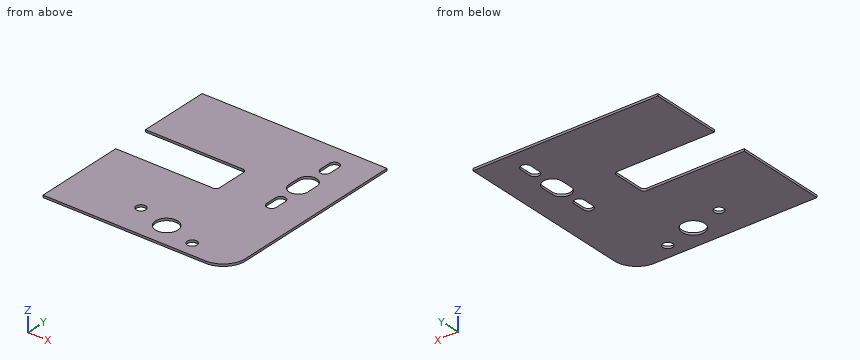
from build123d import *

# Parameters (mm, degrees)
ESQUISSE1_W             = 247
ESQUISSE1_H             = 267
ESQUISSE1_R             = 12.5
ESQUISSE1_R_2           = 6.5
BOSS_EXTRU_1_DEPTH      = 3
ESQUISSE3_R             = 6.5
ESQUISSE3_R_2           = 15
ENL_V_MAT_EXTRU_2_DEPTH = 3
ESQUISSE4_W             = 135
ESQUISSE4_H             = 50
ENL_V_MAT_EXTRU_3_DEPTH = 10
CONG_1_R                = 5
CONG_2_R                = 30
ENL_V_MAT_EXTRU_4_DEPTH = 10


with BuildPart() as part:
    # Esquisse1 → Boss.-Extru.1 (new body)
    with BuildSketch(Plane.XY):
        Rectangle(ESQUISSE1_W, ESQUISSE1_H)
        with Locations((76.5, 51.5)):
            Circle(ESQUISSE1_R, mode=Mode.SUBTRACT)
        with Locations((76.5, 96.5)):
            Circle(ESQUISSE1_R_2, mode=Mode.SUBTRACT)
        with Locations((76.5, 6.5)):
            Circle(ESQUISSE1_R_2, mode=Mode.SUBTRACT)
    extrude(amount=BOSS_EXTRU_1_DEPTH)

    # Esquisse3 → Enlèv. mat.-Extru.2 (cut)
    with BuildSketch(Plane(origin=(0, 0, 0), x_dir=(-1, 0, 0), z_dir=(0, 0, -1))):
        with Locations((-59.966662183, -113.5)):
            Circle(ESQUISSE3_R)
        with Locations((-16.5, -101.85314297)):
            Circle(ESQUISSE3_R_2)
        with Locations((26.966662183, -90.206285941)):
            Circle(ESQUISSE3_R)
    extrude(amount=-ENL_V_MAT_EXTRU_2_DEPTH, mode=Mode.SUBTRACT)

    # Esquisse4 → Enlèv. mat.-Extru.3 (cut)
    with BuildSketch(Plane(origin=(0, 0, 0), x_dir=(-1, 0, 0), z_dir=(0, 0, -1))):
        with Locations((56, 13.5)):
            Rectangle(ESQUISSE4_W, ESQUISSE4_H)
    extrude(amount=-ENL_V_MAT_EXTRU_3_DEPTH, mode=Mode.SUBTRACT)

    # Congé1
    cong_1_edges = [part.edges().sort_by_distance(p)[0] for p in [
        (11.5, -11.5, 1.5),
        (11.5, 38.5, 1.5),
    ]]
    fillet(cong_1_edges, radius=CONG_1_R)

    # Congé2
    cong_2_edges = [part.edges().sort_by_distance(p)[0] for p in [
        (123.5, -133.5, 1.5),
    ]]
    fillet(cong_2_edges, radius=CONG_2_R)

    # Esquisse5 → Enlèv. mat.-Extru.4 (cut)
    with BuildSketch(Plane(origin=(0, 0, 0), x_dir=(-1, 0, 0), z_dir=(0, 0, -1))):
        with BuildLine():
            Line((-83, 89), (-83, 104))
            ThreePointArc((-83, 104), (-76.5, 110.5), (-70, 104))
            Line((-70, 104), (-70, 89))
            ThreePointArc((-70, 89), (-76.5, 82.5), (-83, 89))
        make_face()
        with BuildLine():
            Line((-83, -1), (-83, 14))
            ThreePointArc((-83, 14), (-76.5, 20.5), (-70, 14))
            Line((-70, 14), (-70, -1))
            ThreePointArc((-70, -1), (-76.5, -7.5), (-83, -1))
        make_face()
        with BuildLine():
            Line((-89, 44), (-89, 59))
            ThreePointArc((-89, 59), (-76.5, 71.5), (-64, 59))
            Line((-64, 59), (-64, 44))
            ThreePointArc((-64, 44), (-76.5, 31.5), (-89, 44))
        make_face()
    extrude(amount=-ENL_V_MAT_EXTRU_4_DEPTH, mode=Mode.SUBTRACT)


solid = part.part
Build history of the part. All positions in model axes, mm. Give positions to 0.01 mm unless a question says otherwise; leave off trailing zeros. Order: outer loops, then holes, each group sorted by start corner. A loop starts at its lowest first (then second) coordinate and runs counter-clockwise, first axis right, second up. Notation, with made-up numbers: M 14.5,57.25 L 44.5,57.25 A19 cw 44.5,62.25 Z; hole C 15,23.5 d5. An arc over 180 degrees is marked long. Put each result on its own line as item: value.
Item 1: Slice it at C-C, the plane x = 76.5. Write the cut outline in (y, z), plus the area to 3 significant figures.
From the geometry:
outline: M -133.5,0 L -7.5,0 L -7.5,3 L -133.5,3 Z; M 20.5,0 L 31.5,0 L 31.5,3 L 20.5,3 Z; M 71.5,0 L 82.5,0 L 82.5,3 L 71.5,3 Z; M 110.5,0 L 133.5,0 L 133.5,3 L 110.5,3 Z
area: 513 mm2
Item 2: Flat gauge pins, fed straight in: pin 1 Ø12 at (x, y) = (49.5, -27) entering from -Z; pin 2 Ø0.9 at (y, z) = (21, 1.5) entering from -X. Where does each tip first touch, or does it go through?
From the geometry:
pin 1: stops at z = 0
pin 2: stops at x = 11.5
Item 3: Slice it at A-A, the plane x = -93. Write the cut outline in (y, z), plus the area to 3 significant figures.
From the geometry:
outline: M -133.5,0 L -11.5,0 L -11.5,3 L -133.5,3 Z; M 38.5,0 L 133.5,0 L 133.5,3 L 38.5,3 Z
area: 651 mm2
Item 4: Slice it at B-B, the plane z = 1.55. Write the cut outline in (x, y).
From the geometry:
outline: M -123.5,-133.5 L 93.5,-133.5 A30 ccw 123.5,-103.5 L 123.5,133.5 L -123.5,133.5 L -123.5,38.5 L 6.5,38.5 A5 cw 11.5,33.5 L 11.5,-6.5 A5 cw 6.5,-11.5 L -123.5,-11.5 Z; hole C -26.97,-90.21 d13; hole C 16.5,-101.85 d30; hole C 59.97,-113.5 d13; hole M 64,44 A12.5 ccw 89,44 L 89,59 A12.5 ccw 64,59 Z; hole M 70,-1 A6.5 ccw 83,-1 L 83,14 A6.5 ccw 70,14 Z; hole M 70,89 A6.5 ccw 83,89 L 83,104 A6.5 ccw 70,104 Z
Item 5: Slice it at D-D, the plane y = -113.5. Write the cut outline in (x, z), plus the area to 3 significant figures.
From the geometry:
outline: M -123.5,0 L 7.05,0 L 7.05,3 L -123.5,3 Z; M 25.95,0 L 53.47,0 L 53.47,3 L 25.95,3 Z; M 66.47,0 L 121.78,0 L 121.78,3 L 66.47,3 Z
area: 640 mm2
Item 6: Probe line 1 (X direction, y = 98, z = 0.6); line 2 (Y direction, x = -110, z = 2.55); line 3 (Y direction, x = 16.5, z = 2.8). List the from-to ranges inside material, lowest first. Write a range as [from, to].
From the geometry:
line 1: x = [-123.5, 70], [83, 123.5]
line 2: y = [-133.5, -11.5], [38.5, 133.5]
line 3: y = [-133.5, -116.85], [-86.85, 133.5]
